Source: three-view drawing plus pictorial views. Frame: mm from the lowest corner of the part. Give positions to 0.01 mm unless a question says otherwise; leave off trailing zeros. Order: outer loops, then holes, each group sorted by start corner. A loop starts at its lowest first (then second) coordinate and runs counter-clockwise, first axis right, second up. Notation, with made-up numbers: (-9, 59.5) -> (36, 59.5) arc R27 cw to (36, 93.5) -> close; hole circle Ø6 at (61.25, 40). An arc over 180 degrees is marked (long way). Answer in a Markdown table with one row per item. Add a question column.
Q1. Cut plane B-B on z = 32. Return the cut outline in (x, y), and give its area (3 significant figures).
Q2. Line query: line 1 along Z through (x, y) = (8, 30.5); line 2 along Y through (x, z) = (20, 46); line 3 along Y through (x, z) = (18, 18). Output: solid intervals per line, ascending. Write a range as from..to.
Q3. Cut plane C-C on y = 5. Return the cut outline in (x, z).
Q4. Cut plane A-A on y = 26. Return the cut outline in (x, z), and give its area (3 significant figures).
Q5. Contact query for flat-ended pins moving along their axis: P1, Ø5, axis at x = 24.5, z = 26.5, coming from the +Y side; P2, Ø10, axis at x = 16.5, y = 10, coming from the -Z side; P3, Ø2, axis at x = 40.5, z = 15.5, coming from the +Y side; P4, Ø2, axis at x = 10.5, y = 11.5, coming from the +Z side. Output: stop coordinate, or through.
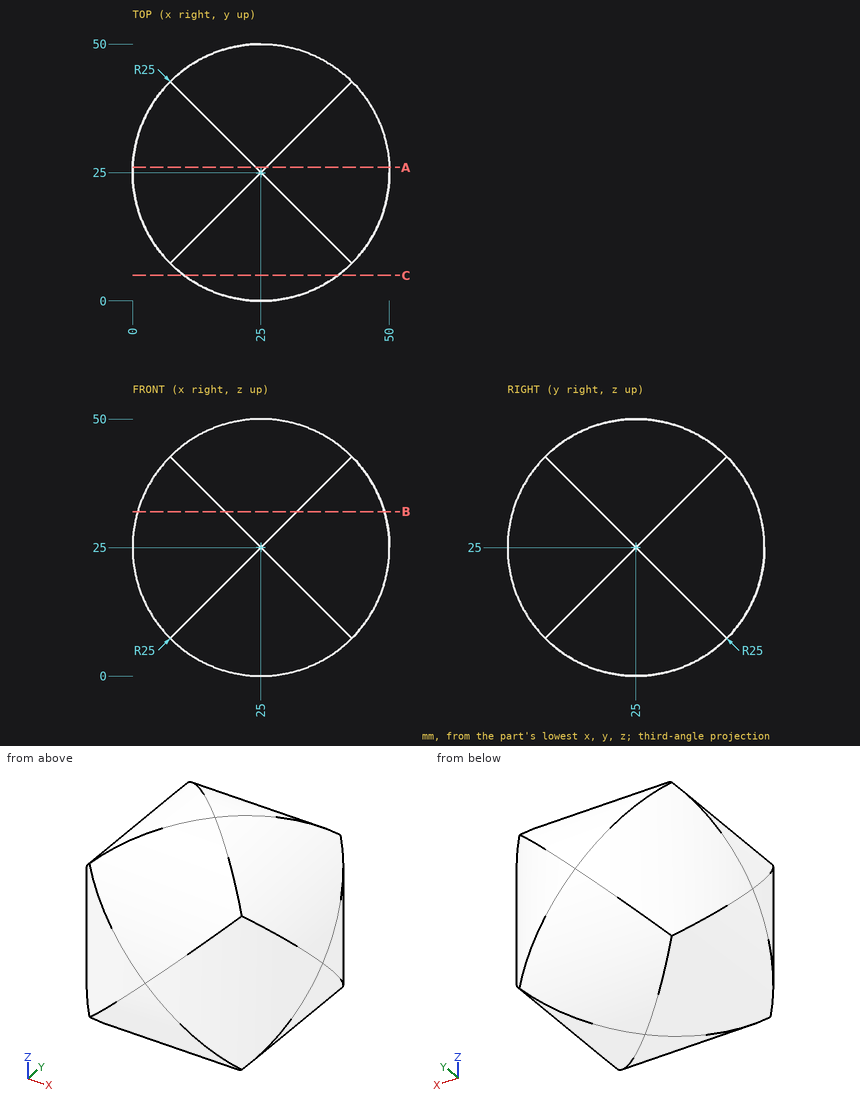
Completed:
| question | item | result |
|---|---|---|
| 1 | outline | (1, 18) arc R25 ccw to (18, 1) -> (32, 1) arc R25 ccw to (49, 18) -> (49, 32) arc R25 ccw to (32, 49) -> (18, 49) arc R25 ccw to (1, 32) -> close |
| 1 | area | 1,930 mm² |
| 2 | line 1 | z = 6.67..43.33 |
| 2 | line 2 | y = 11.44..38.56 |
| 2 | line 3 | y = 1..49 |
| 3 | outline | (10, 10) -> (40, 10) -> (40, 40) -> (10, 40) -> close |
| 4 | outline | (0.02, 24) arc R25 ccw to (24, 0.02) -> (26, 0.02) arc R25 ccw to (49.98, 24) -> (49.98, 26) arc R25 ccw to (26, 49.98) -> (24, 49.98) arc R25 ccw to (0.02, 26) -> close |
| 4 | area | 1,960 mm² |
| 5 | P1 | stops at y = 50 |
| 5 | P2 | stops at z = 2.09 |
| 5 | P3 | stops at y = 45.37 |
| 5 | P4 | stops at z = 46.04 |
